```python
from build123d import *

# Parameters (mm, degrees)
SKETCH_1_W               = 35
SKETCH_1_H               = 70
EXTRUDE_1_DEPTH          = 6
SKETCH_1_W_2             = 26
EXTRUDE_1_2_DEPTH        = 6
SKETCH_1_3_W             = 14
SKETCH_1_3_H             = 70
EXTRUDE_2_DEPTH          = 120
EXTRUDE_4_DEPTH          = 70
EXTRUDE_7_DEPTH          = 70
SKETCH_7_R               = 3
CUT_EXTRUDE_4_DEPTH      = 121
SKETCH_8_R               = 5
CUT_EXTRUDE_5_DEPTH      = 115
SKETCH_3_R               = 11.1
SKETCH_3_R_2             = 4.1
SKETCH_3_R_3             = 2
CUT_EXTRUDE_8_DEPTH      = 36
CUT_EXTRUDE_8_DEPTH_BACK = 41
SKETCH_10_W              = 75
SKETCH_10_H              = 24
EXTRUDE_8_DEPTH          = 6
CUT_EXTRUDE_START        = -6
SKETCH_11_R              = 3
CUT_EXTRUDE_9_DEPTH      = 29
SKETCH_12_W              = 56.46589335
SKETCH_12_H              = 70
CUT_EXTRUDE_10_DEPTH     = 70
FILLET_1_R               = 5
SKETCH_13_R              = 5
CUT_EXTRUDE_11_DEPTH     = 23
SKETCH_14_W              = 75
SKETCH_14_H              = 16
CUT_EXTRUDE_12_DEPTH     = 10
SKETCH_15_R              = 1.5
CUT_EXTRUDE_13_DEPTH     = 6.25
SKETCH_16_R              = 1.5
CUT_EXTRUDE_14_DEPTH     = 6


with BuildPart() as part:
    # Sketch 1 → Extrude 1 (new body)
    with BuildSketch(Plane(origin=(0, 0, 0), x_dir=(1, 0, 0), z_dir=(0, 1, 0))):
        with Locations((17.5, -35)):
            Rectangle(SKETCH_1_W, SKETCH_1_H)
    extrude(amount=EXTRUDE_1_DEPTH)



with BuildPart() as body_2:
    # Sketch 1 → Extrude 1 2 (new body)
    with BuildSketch(Plane(origin=(0, 0, 0), x_dir=(1, 0, 0), z_dir=(0, 1, 0))):
        with Locations((62, -35)):
            Rectangle(SKETCH_1_W_2, SKETCH_1_H)
    extrude(amount=EXTRUDE_1_2_DEPTH)


with BuildPart() as part_1:
    add(part.part)

    add(body_2.part)  # Extrude 2 merges body 2
    # Sketch 1_3 → Extrude 2 (add)
    with BuildSketch(Plane(origin=(0, 0, 0), x_dir=(1, 0, 0), z_dir=(0, 1, 0))):
        with Locations((42, -35)):
            Rectangle(SKETCH_1_3_W, SKETCH_1_3_H)
    extrude(amount=EXTRUDE_2_DEPTH)

    # Sketch 4 → Extrude 4 (add, through all)
    with BuildSketch(Plane(origin=(0, 0, 0), x_dir=(-1, 0, 0), z_dir=(0, 0, -1))):
        Polygon((-35, 6), (-15, 6), (-35, 38), align=None)
        Polygon((-60, 6), (-40, 38), (-40, 6), align=None)
    extrude(amount=-EXTRUDE_4_DEPTH)

    # Sketch 9 → Extrude 7 (add, through all)
    with BuildSketch(Plane(origin=(0, 0, 0), x_dir=(-1, 0, 0), z_dir=(0, 0, -1))):
        Polygon((-35, 120), (-15, 6), (-35, 0), align=None)
    extrude(amount=-EXTRUDE_7_DEPTH)

    # Sketch 7 → Cut-Extrude 4 (cut, through all)
    with BuildSketch(Plane.XZ):
        with Locations((62.5, 47.5)):
            Circle(SKETCH_7_R)
        with Locations((62.5, 22.5)):
            Circle(SKETCH_7_R)
        with Locations((12.5, 22.5)):
            Circle(SKETCH_7_R)
        with Locations((12.5, 47.5)):
            Circle(SKETCH_7_R)
    extrude(amount=-CUT_EXTRUDE_4_DEPTH, mode=Mode.SUBTRACT)

    # Sketch 8 → Cut-Extrude 5 (cut)
    with BuildSketch(Plane(origin=(0, 6, 0), x_dir=(1, 0, 0), z_dir=(0, 1, 0))):
        with Locations((12.5, -47.5)):
            Circle(SKETCH_8_R)
        with Locations((12.5, -22.5)):
            Circle(SKETCH_8_R)
        with Locations((62.5, -47.5)):
            Circle(SKETCH_8_R)
        with Locations((62.5, -22.5)):
            Circle(SKETCH_8_R)
    extrude(amount=CUT_EXTRUDE_5_DEPTH, mode=Mode.SUBTRACT)

    # Sketch 3 → Cut-Extrude 8 (cut, two sides)
    with BuildSketch(Plane.ZY.offset(-35)) as cut_extrude_8_sk:
        with Locations((35, 86)):
            Circle(SKETCH_3_R)
        with Locations((35, 66.75)):
            Circle(SKETCH_3_R_2)
        with Locations((35, 57)):
            Circle(SKETCH_3_R_3)
        with Locations((9.88526329, 100.5)):
            Circle(SKETCH_3_R_3)
        with Locations((60.11473671, 100.5)):
            Circle(SKETCH_3_R_3)
    extrude(amount=CUT_EXTRUDE_8_DEPTH, mode=Mode.SUBTRACT)
    extrude(cut_extrude_8_sk.sketch, amount=-CUT_EXTRUDE_8_DEPTH_BACK, mode=Mode.SUBTRACT)

    # Sketch 10 → Extrude 8 (add)
    with BuildSketch(Plane.XZ):
        with Locations((37.5, 82)):
            Rectangle(SKETCH_10_W, SKETCH_10_H)
    extrude_8 = extrude(amount=-EXTRUDE_8_DEPTH)

    # Sketch 11 → Cut-Extrude 9 (cut)
    with BuildSketch(Plane(origin=(0, 6, 0), x_dir=(1, 0, 0), z_dir=(0, 1, 0)).offset(CUT_EXTRUDE_START)):
        with Locations((37.5, -72.5)):
            Circle(SKETCH_11_R)
    cut_extrude_9 = extrude(amount=CUT_EXTRUDE_9_DEPTH, mode=Mode.SUBTRACT)

    # Mirror 1: Extrude 8, Cut-Extrude 9 across plane
    add(extrude_8.mirror(Plane.XY.offset(35)))
    add(cut_extrude_9.mirror(Plane.XY.offset(35)), mode=Mode.SUBTRACT)

    # Sketch 12 → Cut-Extrude 10 (cut)
    with BuildSketch(Plane(origin=(0, 120, 0), x_dir=(1, 0, 0), z_dir=(0, 1, 0))):
        with Locations((6.767053325, -35)):
            Rectangle(SKETCH_12_W, SKETCH_12_H)
    extrude(amount=-CUT_EXTRUDE_10_DEPTH, mode=Mode.SUBTRACT)

    # Fillet 1
    fillet_1_edges = [part_1.edges().sort_by_distance(p)[0] for p in [
        (22.719298246, 50, 35),
    ]]
    fillet(fillet_1_edges, radius=FILLET_1_R)

    # Sketch 13 → Cut-Extrude 11 (cut)
    with BuildSketch(Plane(origin=(0, 6, 0), x_dir=(1, 0, 0), z_dir=(0, 1, 0))):
        with Locations((37.5, -72.5)):
            Circle(SKETCH_13_R)
        with Locations((37.5, 2.5)):
            Circle(SKETCH_13_R)
    extrude(amount=CUT_EXTRUDE_11_DEPTH, mode=Mode.SUBTRACT)

    # Sketch 14 → Cut-Extrude 12 (cut)
    with BuildSketch(Plane(origin=(0, 6, 0), x_dir=(1, 0, 0), z_dir=(0, 1, 0))):
        with Locations((37.5, 16)):
            Rectangle(SKETCH_14_W, SKETCH_14_H)
        with Locations((37.5, -86)):
            Rectangle(SKETCH_14_W, SKETCH_14_H)
    extrude(amount=-CUT_EXTRUDE_12_DEPTH, mode=Mode.SUBTRACT)

    # Sketch 15 → Cut-Extrude 13 (cut)
    with BuildSketch(Plane(origin=(0, 120, 0), x_dir=(1, 0, 0), z_dir=(0, 1, 0))):
        with Locations((40, -35)):
            Circle(SKETCH_15_R)
    extrude(amount=-CUT_EXTRUDE_13_DEPTH, mode=Mode.SUBTRACT)

    # Sketch 16 → Cut-Extrude 14 (cut)
    with BuildSketch(Plane.ZY.offset(-35)):
        with Locations((35, 115)):
            Circle(SKETCH_16_R)
    extrude(amount=-CUT_EXTRUDE_14_DEPTH, mode=Mode.SUBTRACT)


solid = part_1.part
```
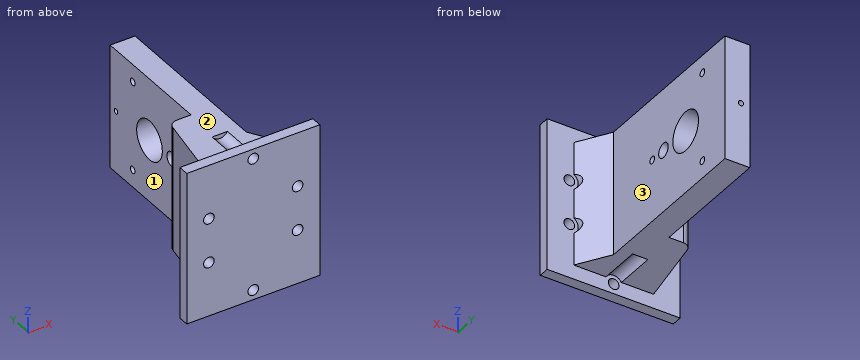
Work out the finished part from the listing and answer in its coordinate system (mm). Face numbers are marked on the shaded views. A direction names the side the tool comes from. Round coordinates to 2 decimals unless told otherwise and drop trailing zeros. Write each loop counter-clockwise with the first axis right and the second up, starting at its lowest first coordinate (ties: lowest second). Pieces come first, ordered by that corner, then holes.
1) A cutting plane is placed at D-D on z = 54. Determine the outline of the cut face in (x, y).
2) Which of the six approach directions +Z, -Z, +X, -X, +Y, -Y give full straight-line access (tool end or side, diameter ignored) to the marked faces 1, 2 and 3?
3) A cutting plane is placed at B-B on x = 12.5. Determine the outline of the cut face in (y, z), and give its area (3 significant figures).
4) Flat-ended cylindrical pins translate along their axes: P1, Ø12, axis at x = 8.5, z = 64.5, coming from the +Y side; P2, Ø10, axis at y = 90, z = 52, coming from the -X side; P3, Ø2, axis at x = 43.5, y = 64.5, coming from the +Z side. Find the tip coordinate at first contact, or state that the pin passes through.
5) A cutting plane is placed at C-C on z = -2.5. Determine the outline of the cut face in (x, y).
6) A cutting plane is placed at A-A on y = 57. Determine the outline of the cut face in (x, z), and give its area (3 significant figures).
7) Consider probe 1 along Y at (x, z) = (42.25, 35); probe 2 along Z at (x, y) = (12.5, 4.5); probe 3 along X at (y, z) = (3.7, 72.5). Determine where each line is inside the solid, lowest interval first.
Entries:
1. outline: (0, 0) - (75, 0) - (75, 6) - (60, 6) - (49, 23.6) - (49, 120) - (35, 120) - (35, 50) - (26.92, 50) arc R5 ccw to (21.99, 45.86) - (15, 6) - (0, 6) - close
2. face 1: +Z, -Z, -X, +Y
2. face 2: +Z, +X, -X, +Y
2. face 3: +Z, -Z, +X, +Y
3. outline: (0, -8) - (6, -8) - (6, 19.5) - (0, 19.5) - close; (0, 25.5) - (6, 25.5) - (6, 44.5) - (0, 44.5) - close; (0, 50.5) - (6, 50.5) - (6, 78) - (0, 78) - close
3. area: 444 mm2
4. P1: stops at y = 6
4. P2: stops at x = 35
4. P3: stops at z = 70
5. outline: (0, 0) - (34.5, 0) - (34.5, 6) - (0, 6) - close; (40.5, 0) - (75, 0) - (75, 6) - (40.5, 6) - close
6. outline: (35, 0) - (49, 0) - (49, 33) - (35, 33) - close; (35, 37) - (49, 37) - (49, 70) - (35, 70) - close
6. area: 924 mm2
7. probe 1: y = 0 to 55, 59 to 62.65, 70.85 to 74.9, 97.1 to 120
7. probe 2: z = -8 to 19.5, 25.5 to 44.5, 50.5 to 78
7. probe 3: x = 0 to 34.5, 40.5 to 75
